Source: CAD feature listing. Evaluate the final solid. Frame: model axes, mm. A direction names the side the tool comes from. Coordinates: 2 decimals unless noted, no trailing zeros. Write each loop counter-clockwise with the first axis right and the second up, starting at its lowest first coordinate (ties: lowest second). Pieces come first, ordered by that corner, then holes. Notation, with made-up numbers: M -3.75,76.5 L 20.25,76.5 A15 cw 20.25,84.5 Z; hole C 7.5,-30 d5. An arc over 180 degrees is marked long. One line per item, written item: value. Start each with the question number.
Item 1: Cut plane C-C, the plane z = -2. Output: boundary loops of the cut face in (x, y).
Item 2: Mould query, pull axis X, two halves, no side actions, for faces 4 (the cylindrical face through (-33.472, 38.551, 0.908)), 5 (the flat face through (0, 35, -53)), 6 (the flat face through (0, 20, -72.5)). Classes: released by +X, released by -X, zero draft, split by the parting line, or undercut.
Item 3: Cut plane D-D, the plane x = 19.5. Output: boundary loops of the cut face in (y, z).
Item 4: Set-up query: faces 1 (the flat face through (-8.33, 41, -6)), 2 (the flat face through (-16, 41, 28.476)), 3 (the flat face through (-16, 41, 55.146)). Return all of +Z, -Z, +X, -X, +Y, -Y with unobstructed straight access to the full face (end or side cutting, diameter ignored); none if empty.
Item 5: Cut plane B-B, the plane x = -5. Output: boundary loops of the cut face in (y, z), then the cut area to 3 significant figures.
Item 6: Ray query, L1, parallel to Y at x = 20.5, z = 29; L2, parallel to Y at x = -16.5, z = -47.5; L3, parallel to Z at x = 15, y = 36.5. Return the intervals inside material, ascending. Write a range as from..to.
Item 7: Cut plane A-A, the plane z = 57. Output: boundary loops of the cut face in (x, y).
Item 8: Pin query (flat end, axial travel): P1, Ø0.8, axis at y = 41.5, z = 48.5, coming from the -X side; P2, Ø3, axis at y = 38, z = 15, coming from the -X side; P3, Ø20.5, axis at x = 14, z = -57.5, coming from the +Y side. Return the tip coordinate at first contact, or that it passes through.
```python
from build123d import *

# Parameters (mm, degrees)
SKETCH1_W           = 70
SKETCH1_H           = 145
BOSS_EXTRUDE1_DEPTH = 40
SKETCH2_W           = 57.3
SKETCH2_H           = 25.847658175
CUT_EXTRUDE1_DEPTH  = 5
SKETCH3_W           = 15.24
SKETCH3_H           = 15.24
BOSS_EXTRUDE2_DEPTH = 2.5
LPATTERN1_COUNT     = 3
LPATTERN1_PITCH     = 26.67
FILLET1_R           = 7.62
FILLET2_R           = 5.08
FILLET3_R           = 5.08


with BuildPart() as part:
    # Sketch1 → Boss-Extrude1 (new body)
    with BuildSketch(Plane(origin=(0, 0, 0), x_dir=(1, 0, 0), z_dir=(0, 1, 0))):
        Rectangle(SKETCH1_W, SKETCH1_H)
    extrude(amount=BOSS_EXTRUDE1_DEPTH)

    # Sketch2 → Cut-Extrude1 (cut)
    with BuildSketch(Plane(origin=(0, 40, 0), x_dir=(1, 0, 0), z_dir=(0, 1, 0))):
        with Locations((0, 53.226170913)):
            Rectangle(SKETCH2_W, SKETCH2_H)
    extrude(amount=-CUT_EXTRUDE1_DEPTH, mode=Mode.SUBTRACT)

    # Sketch3 → Boss-Extrude2 (add)
    with BuildSketch(Plane(origin=(0, 40, 0), x_dir=(1, 0, 0), z_dir=(0, 1, 0))):
        with Locations((-15.95, 5.814113942)):
            Rectangle(SKETCH3_W, SKETCH3_H)
        with Locations((15.95, 5.814113942)):
            Rectangle(SKETCH3_W, SKETCH3_H)
    boss_extrude2 = extrude(amount=BOSS_EXTRUDE2_DEPTH)

    # LPattern1: Boss-Extrude2 ×3
    with Locations(*[(0, 0, i * LPATTERN1_PITCH) for i in range(1, LPATTERN1_COUNT)]):
        add(boss_extrude2)

    # Fillet1
    fillet1_edges = [part.edges().sort_by_distance(p)[0] for p in [
        (35, 20, 72.5),
        (-35, 20, 72.5),
        (-35, 20, -72.5),
        (35, 20, -72.5),
    ]]
    fillet(fillet1_edges, radius=FILLET1_R)

    # Fillet2
    fillet2_edges = [part.edges().sort_by_distance(p)[0] for p in [
        (35, 40, 0),
        (0, 40, 72.5),
        (0, 40, -72.5),
        (-35, 40, 0),
        (32.768153673, 40, -70.268153673),
        (-32.768153673, 40, -70.268153673),
        (-32.768153673, 40, 70.268153673),
        (32.768153673, 40, 70.268153673),
    ]]
    fillet(fillet2_edges, radius=FILLET2_R)

    # Fillet3
    fillet3_edges = [part.edges().sort_by_distance(p)[0] for p in [
        (35, 0, 0),
        (0, 0, 72.5),
        (-35, 0, 0),
        (0, 0, -72.5),
        (32.768153673, 0, -70.268153673),
        (-32.768153673, 0, -70.268153673),
        (-32.768153673, 0, 70.268153673),
        (32.768153673, 0, 70.268153673),
    ]]
    fillet(fillet3_edges, radius=FILLET3_R)


solid = part.part
```
From the geometry:
1. outline: M -35,5.08 A5.08 ccw -29.92,0 L 29.92,0 A5.08 ccw 35,5.08 L 35,34.92 A5.08 ccw 29.92,40 L 23.57,40 L 23.57,42.5 L 8.33,42.5 L 8.33,40 L -8.33,40 L -8.33,42.5 L -23.57,42.5 L -23.57,40 L -29.92,40 A5.08 ccw -35,34.92 Z
2. face 4: released by -X
2. face 5: undercut
2. face 6: zero draft
3. outline: M 0,-67.42 A5.08 ccw 5.08,-72.5 L 34.92,-72.5 A5.08 ccw 40,-67.42 L 40,-66.15 L 35,-66.15 L 35,-40.3 L 40,-40.3 L 40,-13.43 L 42.5,-13.43 L 42.5,1.81 L 40,1.81 L 40,13.24 L 42.5,13.24 L 42.5,28.48 L 40,28.48 L 40,39.91 L 42.5,39.91 L 42.5,55.15 L 40,55.15 L 40,67.42 A5.08 ccw 34.92,72.5 L 5.08,72.5 A5.08 ccw 0,67.42 Z
4. face 1: +Z, -Z, +Y
4. face 2: +X, -X, +Y
4. face 3: +Z, +X, -X, +Y
5. outline: M 0,-67.42 A5.08 ccw 5.08,-72.5 L 34.92,-72.5 A5.08 ccw 40,-67.42 L 40,-66.15 L 35,-66.15 L 35,-40.3 L 40,-40.3 L 40,67.42 A5.08 ccw 34.92,72.5 L 5.08,72.5 A5.08 ccw 0,67.42 Z
5. area: 5,650 mm²
6. L1: y = 0..40
6. L2: y = 0..35
6. L3: z = -72.25..-66.15, -40.3..72.25
7. outline: M -35,5.08 A5.08 ccw -29.92,0 L 29.92,0 A5.08 ccw 35,5.08 L 35,34.92 A5.08 ccw 29.92,40 L -29.92,40 A5.08 ccw -35,34.92 Z
8. P1: stops at x = -23.57
8. P2: stops at x = -34.75
8. P3: stops at y = 40
